```python
from build123d import *

# Parameters (mm, degrees)
SKETCH1_R           = 6.35
BOSS_EXTRUDE1_DEPTH = 12.7
CUT_EXTRUDE2_DEPTH  = 13.7
FILLET1_R           = 12.7
SKETCH4_R           = 12.7
SKETCH4_R_2         = 6.35
BOSS_EXTRUDE2_DEPTH = 6.35
SKETCH2_W           = 27.073872012
SKETCH2_H           = 29.596885175
CUT_EXTRUDE1_DEPTH  = 3.175


with BuildPart() as part:
    # Sketch1 → Boss-Extrude1 (new body)
    with BuildSketch(Plane(origin=(0, 0, 0), x_dir=(1, 0, 0), z_dir=(0, 1, 0))):
        with BuildLine():
            Line((1.339902706, -174.625), (-42.399739587, -174.625))
            ThreePointArc((-42.399739587, -174.625), (-50.754602331, -177.79991886), (-59.131949668, -174.684811669))
            Line((-59.131949668, -174.684811669), (-96.253765638, -142.415309363))
            ThreePointArc((-96.253765638, -142.415309363), (-144.617963608, -71.634466036), (-152.13989844, 13.761341376))
            ThreePointArc((-152.13989844, 13.761341376), (-145.072520944, 18.99854995), (-139.553151074, 12.149262793))
            ThreePointArc((-139.553151074, 12.149262793), (-129.869632709, -52.503000495), (-91.90140484, -105.720472707))
            Line((-91.90140484, -105.720472707), (-48.88478864, -143.114246675))
            ThreePointArc((-48.88478864, -143.114246675), (-33.347524936, -152.357947214), (-15.556989968, -155.575))
            Line((-15.556989968, -155.575), (1.339902706, -155.575))
            ThreePointArc((1.339902706, -155.575), (10.864902706, -165.1), (1.339902706, -174.625))
        make_face()
        with Locations((-50.8, -165.1)):
            Circle(SKETCH1_R, mode=Mode.SUBTRACT)
        with BuildLine():
            Line((0, -161.925), (1.339902706, -161.925))
            ThreePointArc((1.339902706, -161.925), (4.514902706, -165.1), (1.339902706, -168.275))
            Line((1.339902706, -168.275), (0, -168.275))
            ThreePointArc((0, -168.275), (-3.175, -165.1), (0, -161.925))
        make_face(mode=Mode.SUBTRACT)
    extrude(amount=BOSS_EXTRUDE1_DEPTH)

    # Sketch3 → Cut-Extrude2 (cut, through all)
    with BuildSketch(Plane(origin=(0, 12.7, 0), x_dir=(1, 0, 0), z_dir=(0, 1, 0))):
        with BuildLine():
            Line((-64.278893585, -138.146187914), (-96.067379674, -110.512878542))
            ThreePointArc((-96.067379674, -110.512878542), (-104.093661598, -102.988093371), (-111.532318829, -94.88192461))
            ThreePointArc((-111.532318829, -94.88192461), (-120.588765116, -93.847414192), (-122.222718656, -102.815113283))
            ThreePointArc((-122.222718656, -102.815113283), (-108.389889378, -121.287896312), (-92.087790804, -137.622903528))
            Line((-92.087790804, -137.622903528), (-75.989121055, -151.617263638))
            ThreePointArc((-75.989121055, -151.617263638), (-63.398469458, -150.736839511), (-64.278893585, -138.146187914))
        make_face()
        with BuildLine():
            ThreePointArc((-122.168303836, -80.727586976), (-124.013598755, -88.474110491), (-131.62448434, -86.131428157))
            ThreePointArc((-131.62448434, -86.131428157), (-143.140144863, -54.755391727), (-148.016867664, -21.690551276))
            ThreePointArc((-148.016867664, -21.690551276), (-146.581764091, -20.040770563), (-144.860415421, -21.389198324))
            ThreePointArc((-144.860415421, -21.389198324), (-136.771142128, -52.303847297), (-122.168303836, -80.727586976))
        make_face()
    extrude(amount=-CUT_EXTRUDE2_DEPTH, mode=Mode.SUBTRACT)

    # Fillet1
    fillet1_edges = [part.edges().sort_by_distance(p)[0] for p in [
        (-42.399739587, 6.35, 174.625),
    ]]
    fillet(fillet1_edges, radius=FILLET1_R)

    # Sketch4 → Boss-Extrude2 (add)
    with BuildSketch(Plane(origin=(0, 12.7, 0), x_dir=(1, 0, 0), z_dir=(0, 1, 0))):
        with Locations((-50.8, -165.1)):
            Circle(SKETCH4_R)
        with Locations((-50.8, -165.1)):
            Circle(SKETCH4_R_2, mode=Mode.SUBTRACT)
    extrude(amount=BOSS_EXTRUDE2_DEPTH)

    # Sketch2 → Cut-Extrude1 (cut)
    with BuildSketch(Plane(origin=(0, 12.7, 0), x_dir=(1, 0, 0), z_dir=(0, 1, 0))):
        with Locations((4.011936006, -165.256904056)):
            Rectangle(SKETCH2_W, SKETCH2_H)
    extrude(amount=-CUT_EXTRUDE1_DEPTH, mode=Mode.SUBTRACT)


solid = part.part
```
Check sheet for the modelled part. Datum: model origin and axes. Units: mm. A direction names the side the tool comes from. Round coordinates to 2 decimals unless told otherwise and drop trailing zeros. Write each loop counter-clockwise with the first axis right and the second up, starting at its lowest first coordinate (ties: lowest second). Pieces come first, ordered by that corner, then holes. Notation, with made-up numbers: M 51.5,-38.5 L 90.5,-38.5 A14 cw 90.5,-15.5 Z; hole C -10.5,59.5 d3. An arc over 180 degrees is marked long. Write item = value, one per line. Start each with the question number.
1. Section check C-C, the plane z = 76. Record the cut outline in (x, y), then the cut area to 3 significant figures.
2. Tool access check on faces 1 (the flat face through (-77.43, 6.26, 158.78)), 2 (the cylindrical face through (4.514, 4.696, 165.03)), 3 (the flat face through (-7, 5, 155.575)). Record the directions out of +Z, -Z, +X, -X, +Y, -Y that give a thin tool (end or side, any length) a straight path to the whole face; none if there is none.
3. Gauge pin test, flat ends, axial feed: pin 1 (2 mm diameter, centred on x = -30.5, y = 15, fed in from -Z); pin 2 (6 mm diameter, centred on x = -23.5, y = 8.5, fed in from +Z) (3 decimals); pin 3 (5.5 mm diameter, centred on x = -0.5, z = 163.5, fed in from +Y) (3 decimals); pin 4 (10 mm diameter, centred on x = -122, z = 62.5, fed in from +Y). Record the tip position at first contact, or that the pin passes through.
4. Scan lines: line 1 (Z direction, x = -50.8, y = 14.5); line 2 (X direction, y = 4.5, z = 165.1) (3 decimals); line 3 (X direction, y = 13, z = 165.1). Record each from-to range of solid material in increasing order. Write a range as [from, to].
5. Section check B-B, the plane z = 49. Record the cut outline in (x, y), then the cut area to 3 significant figures.
6. Section check A-A, the plane z = 165.1. Record the cut outline in (x, y) (3 decimals).
7. Release check for a two-part mould opening along X. For faces 4 (the flat face through (-79.951, 6.439, 124.523)), 5 (the cylindrical face through (-144.205, 6.261, 72.775)), 6 (the cylindrical face through (-130.21, 6.26, 51.65)), 7 (the flat face through (-18, 6, 174.625)) record: pulls with the +X half, pulls with the -X half, needs draft (parallel to the pull), parting line crosses it, or undercut.
Results found:
q1.outline = M -142.99,0 L -136.15,0 L -136.15,12.7 L -142.99,12.7 Z; M -125.16,0 L -117.67,0 L -117.67,12.7 L -125.16,12.7 Z
q1.area = 182 mm^2
q2.face_1 = +Z, -X, +Y, -Y
q2.face_2 = +Y, -Y
q2.face_3 = -Z, +X, +Y, -Y
q3.pin_1 = through
q3.pin_2 = 174.625
q3.pin_3 = 9.525
q3.pin_4 = 12.7
q4.line_1 = [152.4, 158.75], [171.45, 177.8]
q4.line_2 = [-70.158, -57.15], [-44.45, -3.175], [4.515, 10.865]
q4.line_3 = [-63.5, -57.15], [-44.45, -38.1]
q5.outline = M -150.98,0 L -144.49,0 L -144.49,12.7 L -150.98,12.7 Z; M -137.99,0 L -131.23,0 L -131.23,12.7 L -137.99,12.7 Z
q5.area = 168 mm^2
q6.outline = M -70.158,0 L -57.15,0 L -57.15,19.05 L -63.5,19.05 L -63.5,12.7 L -70.158,12.7 Z; M -44.45,0 L -3.175,0 L -3.175,9.525 L -9.525,9.525 L -9.525,12.7 L -38.1,12.7 L -38.1,19.05 L -44.45,19.05 Z; M 4.515,0 L 10.865,0 L 10.865,9.525 L 4.515,9.525 Z
q7.face_4 = undercut
q7.face_5 = pulls with the -X half
q7.face_6 = pulls with the +X half
q7.face_7 = needs draft
